Input: part model. Units: mm. Frame: model coordinates. Face numbers are marked on the shaded views. A direction names the side the tool comes from. Round coordinates to 2 decimals unless told otherwise and drop trailing zeros. Write each loop counter-clockwise with the first axis right and the second up, starting at its lowest first coordinate (ties: lowest second). Pieces come first, ordered by that corner, then holes. Notation, with made-up numbers: (81, -4.5) - (134, -4.5) arc R26 ccw to (134, 21.5) - close; hole circle Ø1 at (43.5, -24.75). An arc over 180 degrees is marked (long way). One line per item, written item: value. Start each with the question number.
```python
from build123d import *

# Parameters (mm, degrees)
AUFSATZ_LINEAR_AUSTRAGEN1_DEPTH                      = 10
F_5_4_5_4_DURCHMESSER_LANGLOCH4_DEPTH                = 10
SCHNITT_LINEAR_AUSTRAGEN1_DEPTH                      = 94.789655764
VERRUNDUNG1_R                                        = 3
M4_GEWINDEBOHRUNG2_D                                 = 3.3
M4_GEWINDEBOHRUNG2_DEPTH                             = 11.5
M4_GEWINDEBOHRUNG2_TIP                               = 0.991420021
FORMSENKUNG_F_R_M3_SENKSCHRAUBE_MIT_SCHL_D           = 3.2
FORMSENKUNG_F_R_M3_SENKSCHRAUBE_MIT_SCHL_CSINK_D     = 6.3
FORMSENKUNG_F_R_M3_SENKSCHRAUBE_MIT_SCHL_CSINK_ANGLE = 90
M4_GEWINDEBOHRUNG1_D                                 = 3.3
M4_GEWINDEBOHRUNG1_DEPTH                             = 11.5
M4_GEWINDEBOHRUNG1_TIP                               = 0.991420021
VERRUNDUNG2_R                                        = 10
SKIZZE13_W                                           = 29
SKIZZE13_H                                           = 58
SCHNITT_LINEAR_AUSTRAGEN2_DEPTH                      = 2
FORMSENKUNG_F_R_M3_LINSENSENKSCHRAUBE_MI_D           = 3.4
FORMSENKUNG_F_R_M3_LINSENSENKSCHRAUBE_MI_CSINK_D     = 6.3
FORMSENKUNG_F_R_M3_LINSENSENKSCHRAUBE_MI_CSINK_ANGLE = 90
M4_GEWINDEBOHRUNG3_D                                 = 3.3
M4_GEWINDEBOHRUNG3_DEPTH                             = 11.5
M4_GEWINDEBOHRUNG3_CSINK_D                           = 4.05
M4_GEWINDEBOHRUNG3_CSINK_ANGLE                       = 90
M4_GEWINDEBOHRUNG3_TIP                               = 0.991420021


# Read off the part's stored shape, not the designer's step: Ø5.4 (5.4) Durchmesser Langloch4
with BuildPart() as part:
    # Skizze1 → Aufsatz-Linear austragen1 (new body)
    with BuildSketch(Plane.XY):
        Polygon((28.788534666, -29), (-13.211465334, -4), (-46.211465334, -4), (-46.211465334, 81), (-16.211465334, 81), (-16.211465334, 29), (43.788534666, 29), (43.788534666, -29), align=None)
    extrude(amount=AUFSATZ_LINEAR_AUSTRAGEN1_DEPTH)

    # Ø5.4 (5.4) Durchmesser Langloch4 outline → Ø5.4 (5.4) Durchmesser Langloch4 (cut)
    with BuildSketch(Plane.XY):
        with BuildLine():
            Line((32.488534666, -18.2), (35.088534666, -18.2))
            ThreePointArc((35.088534666, -18.2), (37.788534666, -15.5), (35.088534666, -12.8))
            Line((35.088534666, -12.8), (32.488534666, -12.8))
            ThreePointArc((32.488534666, -12.8), (29.788534666, -15.5), (32.488534666, -18.2))
        make_face()
        with BuildLine():
            Line((32.488534666, 12.8), (35.088534666, 12.8))
            ThreePointArc((35.088534666, 12.8), (37.788534666, 15.5), (35.088534666, 18.2))
            Line((35.088534666, 18.2), (32.488534666, 18.2))
            ThreePointArc((32.488534666, 18.2), (29.788534666, 15.5), (32.488534666, 12.8))
        make_face()
    extrude(amount=F_5_4_5_4_DURCHMESSER_LANGLOCH4_DEPTH, mode=Mode.SUBTRACT)

    # Skizze5 → Schnitt-Linear austragen1 (cut, through all)
    with BuildSketch(Plane(origin=(0, 0, 0), x_dir=(-1, 0, 0), z_dir=(0, 0, -1))):
        Polygon((-23.788534666, -16.713829021), (-23.788534666, 21), (-7.212762179, -6.847297779), align=None)
        Polygon((13.211465334, 21), (13.211465334, 5.309980503), (-0.338419104, -2.7554269), (-14.478554163, 21), align=None)
    extrude(amount=-SCHNITT_LINEAR_AUSTRAGEN1_DEPTH, mode=Mode.SUBTRACT)

    # Verrundung1
    verrundung1_edges = [part.edges().sort_by_distance(p)[0] for p in [
        (7.212762179, -6.847297779, 5),
        (23.788534666, -16.713829021, 5),
        (23.788534666, 21, 5),
        (0.338419104, -2.7554269, 5),
        (14.478554163, 21, 5),
        (-13.211465334, 21, 5),
        (-13.211465334, 5.309980503, 5),
    ]]
    fillet(verrundung1_edges, radius=VERRUNDUNG1_R)

    # M4 Gewindebohrung2
    with Locations(Plane(origin=(0, -4, 0), x_dir=(-1, 0, 0), z_dir=(0, -1, 0))):
        with Locations((23.211465334, -5), (39.211465334, -5)):
            Hole(M4_GEWINDEBOHRUNG2_D / 2, depth=M4_GEWINDEBOHRUNG2_DEPTH)
            with Locations((0, 0, -(M4_GEWINDEBOHRUNG2_DEPTH + M4_GEWINDEBOHRUNG2_TIP / 2))):  # 118° drill point
                Cone(0, M4_GEWINDEBOHRUNG2_D / 2, M4_GEWINDEBOHRUNG2_TIP, mode=Mode.SUBTRACT)

    # Formsenkung für M3 Senkschraube mit Schlitz/Kreuzschlitz1 (through all)
    with Locations(Plane(origin=(0, 0, 0), x_dir=(1, 0, 0), z_dir=(0, 0, -1))):
        with Locations((-31.211465334, -15), (-31.211465334, -1), (-31.211465334, -74), (-31.211465334, -60)):
            CounterSinkHole(FORMSENKUNG_F_R_M3_SENKSCHRAUBE_MIT_SCHL_D / 2, FORMSENKUNG_F_R_M3_SENKSCHRAUBE_MIT_SCHL_CSINK_D / 2, counter_sink_angle=FORMSENKUNG_F_R_M3_SENKSCHRAUBE_MIT_SCHL_CSINK_ANGLE)

    # M4 Gewindebohrung1
    with Locations(Plane(origin=(0, 81, 0), x_dir=(1, 0, 0), z_dir=(0, 1, 0))):
        with Locations((-39.211465334, -5), (-23.211465334, -5)):
            Hole(M4_GEWINDEBOHRUNG1_D / 2, depth=M4_GEWINDEBOHRUNG1_DEPTH)
            with Locations((0, 0, -(M4_GEWINDEBOHRUNG1_DEPTH + M4_GEWINDEBOHRUNG1_TIP / 2))):  # 118° drill point
                Cone(0, M4_GEWINDEBOHRUNG1_D / 2, M4_GEWINDEBOHRUNG1_TIP, mode=Mode.SUBTRACT)

    # Verrundung2
    verrundung2_edges = [part.edges().sort_by_distance(p)[0] for p in [
        (-13.211465334, -4, 5),
        (-16.211465334, 29, 5),
    ]]
    fillet(verrundung2_edges, radius=VERRUNDUNG2_R)

    # Skizze13 → Schnitt-Linear austragen2 (cut)
    with BuildSketch(Plane.XY.offset(10)):
        with Locations((29.288534666, 0)):
            Rectangle(SKIZZE13_W, SKIZZE13_H)
    extrude(amount=-SCHNITT_LINEAR_AUSTRAGEN2_DEPTH, mode=Mode.SUBTRACT)

    # Formsenkung für M3 Linsensenkschraube mit Schlitz1 (through all)
    with Locations(Plane(origin=(0, 0, 0), x_dir=(-1, 0, 0), z_dir=(0, 0, -1))):
        with Locations((21.211465334, 66.5), (21.211465334, 51.5), (41.211465334, 66.5), (41.211465334, 51.5), (21.211465334, 25.5), (21.211465334, 10.5), (41.211465334, 25.5), (41.211465334, 10.5)):
            CounterSinkHole(FORMSENKUNG_F_R_M3_LINSENSENKSCHRAUBE_MI_D / 2, FORMSENKUNG_F_R_M3_LINSENSENKSCHRAUBE_MI_CSINK_D / 2, counter_sink_angle=FORMSENKUNG_F_R_M3_LINSENSENKSCHRAUBE_MI_CSINK_ANGLE)

    # M4 Gewindebohrung3
    with Locations(Plane.ZY.offset(46.211465334)):
        with Locations((5, 39), (5, 18), (5, 60)):
            CounterSinkHole(M4_GEWINDEBOHRUNG3_D / 2, M4_GEWINDEBOHRUNG3_CSINK_D / 2, depth=M4_GEWINDEBOHRUNG3_DEPTH, counter_sink_angle=M4_GEWINDEBOHRUNG3_CSINK_ANGLE)
            with Locations((0, 0, -(M4_GEWINDEBOHRUNG3_DEPTH + M4_GEWINDEBOHRUNG3_TIP / 2))):  # 118° drill point
                Cone(0, M4_GEWINDEBOHRUNG3_D / 2, M4_GEWINDEBOHRUNG3_TIP, mode=Mode.SUBTRACT)


solid = part.part
```
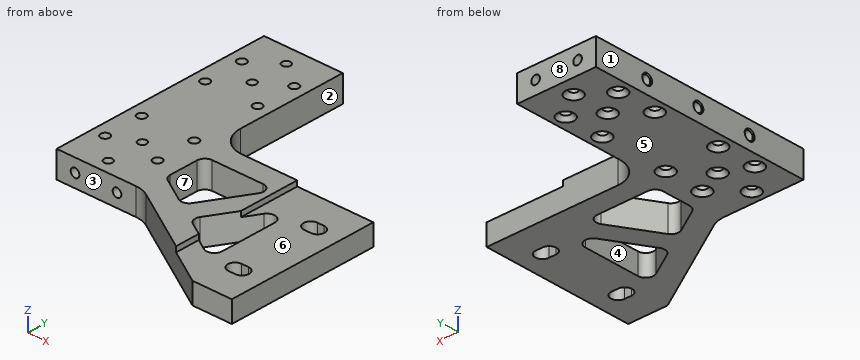
Q1. Cut plane B-B, the plane y = 1. Output: boundary loops of the cut face in (x, z), and give its area (3 significant figures).
Q2. Material intervals for probe 1 along X at (y, z) = (25.5, 6.25); probe 2 along X at (y, z) = (27, 0.75); probe 3 along Y at (x, z) = (-32, 9), sorted ascending. Write a range as from..to.
Q3. Cut plane D-D, the plane x = -3.5. Output: boundary loops of the cut face in (y, z), and give its area (3 significant figures).
Q4. Cut plane C-C, the plane x = 22.5. Output: boundary loops of the cut face in (y, z).
Q5. Access query for the marked faces 1, 2, 3, 4 and 5. Directions: +Z, -Z, +X, -X, +Y, -Y. A direction counts if a zero-diameter tool reaches every point of the face in a straight line with its end or side. Return the directions, or none.
Q6. Contact query for flat-ended pins moving along their axis: pin 1 Ø4 at (x, y) = (-21.21, 10.5) entering from +Z; pin 2 Ø2 at (x, y) = (22.5, 13) entering from +Z; pin 3 Ø2.5 at (x, y) = (-31.21, 1) entering from +Z; pin 4 Ø4 at (y, z) = (60, 5) entering from +X. Output: stop coordinate, or through.
Q7. Cut plane A-A, the plane y = 25.5. Output: boundary loops of the cut face in (x, z).
Q8. Pull-direction query (Y, two-part tool) for the marked faces 6, 7 and 8; classes: pulls with the +Y half, pulls with the -Y half, needs draft (parallel to the pull), parting line crosses it, or undercut.
A:
1. outline: (-46.21, 0) - (-34.36, 0) - (-32.81, 1.55) - (-32.81, 10) - (-46.21, 10) - close; (-29.61, 1.55) - (-28.06, 0) - (-5.97, 0) - (-5.97, 10) - (-29.61, 10) - close; (2.57, 0) - (11.88, 0) - (11.88, 10) - (2.57, 10) - close; (23.79, 0) - (43.79, 0) - (43.79, 8) - (23.79, 8) - close; hole circle Ø3.3 at (-39.21, 5); hole circle Ø3.3 at (-23.21, 5)
1. area: 604 mm²
2. probe 1: x = -46.21..-42.91, -39.51..-22.91, -19.51..43.79
2. probe 2: x = -46.21..-43.08, -39.34..-23.08, -19.34..43.79
2. probe 3: y = -4..-0.39, 2.39..13.61, 16.39..58.61, 61.39..72.61, 75.39..81
3. outline: (-9.78, 0) - (-0.47, 0) - (-0.47, 10) - (-9.78, 10) - close; (21, 0) - (29, 0) - (29, 10) - (21, 10) - close
3. area: 173 mm²
4. outline: (-25.26, 0) - (-13.9, 0) - (-13.9, 8) - (-25.26, 8) - close; (12.56, 0) - (29, 0) - (29, 8) - (12.56, 8) - close
5. face 1: +Z, -Z, -X, +Y, -Y
5. face 2: +Z, -Z, +X, +Y
5. face 3: +Z, -Z, -X, -Y
5. face 4: +Z, -Z
5. face 5: -Z, +X, -X, +Y, -Y
6. pin 1: stops at z = 10
6. pin 2: stops at z = 8
6. pin 3: passes through
6. pin 4: stops at x = -16.21
7. outline: (-46.21, 0) - (-44.36, 0) - (-42.91, 1.45) - (-42.91, 10) - (-46.21, 10) - close; (-39.51, 1.45) - (-38.06, 0) - (-24.36, 0) - (-22.91, 1.45) - (-22.91, 10) - (-39.51, 10) - close; (-19.51, 1.45) - (-18.06, 0) - (43.79, 0) - (43.79, 8) - (14.79, 8) - (14.79, 10) - (-19.51, 10) - close
8. face 6: needs draft
8. face 7: undercut
8. face 8: pulls with the +Y half
